from build123d import *

# Parameters (mm, degrees)
F0_W     = 100
F0_H     = 30
F1_DEPTH = 50
F2_W     = 70
F2_H     = 15
F3_DEPTH = 30
F4_R     = 3.5
F5_DEPTH = 15


with BuildPart() as f1:
    # F0 (on Top) → F1 (new body)
    with BuildSketch(Plane.XY):
        Rectangle(F0_W, F0_H)
    extrude(amount=F1_DEPTH)

    # F2 (on face) → F3 (cut)
    with BuildSketch(Plane.XY.offset(50)):
        Rectangle(F2_W, F2_H)
    extrude(amount=-F3_DEPTH, mode=Mode.SUBTRACT)

    # F4 (on face) → F5 (join)
    with BuildSketch(Plane.XY.offset(20)):
        with Locations((-1.711591, 0)):
            Circle(F4_R)
        with Locations((29, 0)):
            Circle(F4_R)
        with Locations((-29, 0)):
            Circle(F4_R)
    extrude(amount=F5_DEPTH)


solid = f1.part
Read the model definition and answer for the solid it produces. Units are mm, in the model's axes. A direction names the side the tool comes from. Coordinates: 2 decimals unless noted, no trailing zeros. Loops run counter-clockwise (first coordinate to the right, second up) from the corner with the lowest first, then second, coordinate; pieces in that order, holes last.
Q1. Consider probe 1 along X at (y, z) = (-1, 38.5); probe 2 along Y at (x, z) = (14, 46); probe 3 along X at (y, z) = (2.25, 29.5). Determine where each line is inside the solid, lowest interval first.
Q2. The part is cut by section D-D on x = 9. Write down the section's boundary in (y, z), and give its area (3 significant figures).
Q3. The part is cut by section B-B on x = 29. Write down the section's boundary in (y, z).
Q4. The mould has two halves that part along Y. Classify faces 3 (the face through (-1, 15, 25)), 4 (the face through (1.52, -1.34, 27.4)), 5 (the face through (50, 0, 25)): +Y half, -Y half, draft (parallel to the pull), parting line (faces both ways), or undercut.
Q5. Each of these flat-tipped pins is pushed along its axis until it touches: pin 1 Ø2 at (x, y) = (30, 1.5) entering from +Z; pin 2 Ø16.5 at (x, y) = (3.5, -3) entering from +Z. Where does it stop, or does it pass through?
Q6. The part is cut by section A-A on z = 43.5. Write down the section's boundary in (x, y), and give its area (3 significant figures).
Q7. The part is cut by section C-C on y = 0. Write down the section's boundary in (x, z), and give its area (4 significant figures).
Q8. Which of the six approach directions +Z, -Z, +X, -X, +Y, -Y give full straight-line access (tool end or side, diameter ignored) to faces 1 (the face through (-1, -15, 25)), 2 (the face through (-35, 0, 35))?
Results below:
1. probe 1: x = -50 to -35, 35 to 50
1. probe 2: y = -15 to -7.5, 7.5 to 15
1. probe 3: x = -50 to -35, -31.68 to -26.32, -4.39 to 0.97, 26.32 to 31.68, 35 to 50
2. outline: (-15, 0) - (15, 0) - (15, 50) - (7.5, 50) - (7.5, 20) - (-7.5, 20) - (-7.5, 50) - (-15, 50) - close
2. area: 1,050 mm2
3. outline: (-15, 0) - (15, 0) - (15, 50) - (7.5, 50) - (7.5, 20) - (3.5, 20) - (3.5, 35) - (-3.5, 35) - (-3.5, 20) - (-7.5, 20) - (-7.5, 50) - (-15, 50) - close
4. face 3: +Y half
4. face 4: undercut
4. face 5: draft
5. pin 1: stops at z = 35
5. pin 2: stops at z = 50
6. outline: (-50, -15) - (50, -15) - (50, 15) - (-50, 15) - close; hole (-35, -7.5) - (35, -7.5) - (35, 7.5) - (-35, 7.5) - close
6. area: 1,950 mm2
7. outline: (-50, 0) - (50, 0) - (50, 50) - (35, 50) - (35, 20) - (32.5, 20) - (32.5, 35) - (25.5, 35) - (25.5, 20) - (1.79, 20) - (1.79, 35) - (-5.21, 35) - (-5.21, 20) - (-25.5, 20) - (-25.5, 35) - (-32.5, 35) - (-32.5, 20) - (-35, 20) - (-35, 50) - (-50, 50) - close
7. area: 3,215 mm2
8. face 1: +Z, -Z, +X, -X, -Y
8. face 2: +Z
